Autodesk Inventor part; units mm, degrees
ref_plane "YZ Plane" through (0, 0, 0) normal (1, 0, 0) x (0, 1, 0)
ref_plane "XZ Plane" through (0, 0, 0) normal (0, 1, 0) x (-1, 0, 0)
ref_plane "XY Plane" through (0, 0, 0) normal (0, 0, 1) x (1, 0, 0)
sketch "Sketch1" plane through (0, 0, 0) normal (0, 0, 1) x (1, 0, 0)
  line L0 (0, 0) -> (160, 0)
  line L1 (160, 0) -> (118.589, -154.5481) construction
  line L2 (0, 0) -> (41.411, -154.5481) construction
  line L3 (41.411, -154.5481) -> (118.589, -154.5481)
  circle A0 centre (235.8871, -103.156) radius 80 construction
  line L4 (160, 0) -> (256.5926, -25.8819)
  line L5 (118.589, -154.5481) -> (215.1815, -180.43)
  arc A1 (215.1815, -180.43) -> (256.5926, -25.8819) centre (235.8871, -103.156) ccw
  circle A2 centre (-75.8871, -103.156) radius 80 construction
  line L6 (0, 0) -> (-96.5926, -25.8819)
  line L7 (41.411, -154.5481) -> (-55.1815, -180.43)
  arc A3 (-96.5926, -25.8819) -> (-55.1815, -180.43) centre (-75.8871, -103.156) ccw
  dimension "d0" = 160
  dimension "d1" = 160
  dimension "d2" = 160
  dimension "d3" = 75
  dimension "d4" = 75
  dimension "d5" = 160
  dimension "d6" = 100
  dimension "d7" = 160
  dimension "d9" = 100
extrude "Extrusion1" add sketch "Sketch1" along normal blind 41.5
sketch "Sketch2" plane through (0, 0, 41.5) normal (0, 0, 1) x (1, 0, 0)
  line L0 (-26.5, -133) -> (186.5, -133)
  line L1 (186.5, -133) -> (186.5, -20)
  line L2 (186.5, -20) -> (-26.5, -20)
  line L3 (-26.5, -20) -> (-26.5, -133)
  line L4 (160, 0) -> (0, 0)
  point P0 (80, -20)
  point P1 (80, 0)
  dimension "d12" = 213
  dimension "d13" = 113
  dimension "d14" = 20
extrude "Extrusion2" cut sketch "Sketch2" against normal through all
sketch "Sketch3" plane through (0, 0, 41.5) normal (0, 0, 1) x (1, 0, 0)
  line L0 (-26.5, -133) -> (-26.5, -20) construction
  line L1 (-26.5, -20) -> (186.5, -20) construction
  line L2 (186.5, -20) -> (186.5, -133) construction
  line L3 (186.5, -133) -> (-26.5, -133) construction
  line L4 (-48.0481, 1.5481) -> (-48.0481, -154.5481) construction
  line L5 (-48.0481, -154.5481) -> (208.0481, -154.5481) construction
  line L6 (208.0481, -154.5481) -> (208.0481, 1.5481) construction
  line L7 (208.0481, 1.5481) -> (-48.0481, 1.5481) construction
  line L8 (41.411, -154.5481) -> (118.589, -154.5481) construction
  line L9 (-48.0481, 1.5481) -> (-48.0481, -178.5186) construction
  line L10 (-55.1815, -180.43) -> (41.411, -154.5481) construction
  line L11 (208.0481, 1.5481) -> (208.0481, -178.5186) construction
  line L12 (118.589, -154.5481) -> (215.1815, -180.43) construction
  line L13 (-48.0481, -178.5186) -> (208.0481, -178.5186) construction
  line L14 (-48.0481, 1.5481) -> (208.0481, 1.5481) construction
  line L15 (160, 0) -> (256.5926, -25.8819) construction
  line L16 (208.2963, -12.941) -> (208.0481, -178.5186)
  line L17 (208.2963, -12.941) -> (256.5926, -25.8819)
  line L18 (208.0481, -178.5186) -> (215.1815, -180.43)
  arc A0 (215.1815, -180.43) -> (256.5926, -25.8819) centre (235.8871, -103.156) ccw
  line L19 (208.0481, 1.5481) -> (-166.9519, 1.5481)
  line L20 (-166.9519, 1.5481) -> (-166.9519, -188.4519)
  line L21 (-166.9519, -188.4519) -> (208.0481, -188.4519)
  line L22 (208.0481, -188.4519) -> (208.0481, 1.5481)
  point P0 (0, 0)
  point P1 (80, -154.5481)
  dimension "d17" = 190
  dimension "d18" = 375
extrude "Extrusion3" cut sketch "Sketch3" against normal through all contours L22 L21 L20 L19
sketch "Sketch4" plane through (0, 0, 41.5) normal (0, 0, 1) x (1, 0, 0)
  arc A0 (215.1815, -180.43) -> (256.5926, -25.8819) centre (235.8871, -103.156) ccw
  circle A1 centre (235.8871, -103.156) radius 7
  point P0 (0, 0)
  dimension "d21" = 14
extrude "Extrusion4" cut sketch "Sketch4" against normal through all
sketch "Sketch5" plane through (208.0481, -178.5186, 41.5) normal (-1, 0, 0) x (0, 0, 1)
  line L0 (-41.5, 165.6442) -> (0, 165.6442)
  line L1 (-41.5, 0) -> (-41.5, 165.6442)
  line L2 (0, 0) -> (-41.5, 0)
  line L3 (0, 165.6442) -> (0, 0)
  line L4 (-33, 157.1442) -> (-8.5, 157.1442)
  line L5 (-8.5, 157.1442) -> (-8.5, 8.5)
  line L6 (-8.5, 8.5) -> (-33, 8.5)
  line L7 (-33, 8.5) -> (-33, 157.1442)
  point P0 (-41.5, 178.5186)
  dimension "d24" = 8.5
extrude "Extrusion5" add sketch "Sketch5" along normal blind 13 contours L4 L5 L6 L7
sketch "Sketch6" plane through (208.0481, -170.0186, 8.5) normal (0, 0, -1) x (-1, 0, 0)
  circle A0 centre (8, 74.3221) radius 2.5
  line L0 (0, -8.5) -> (0, 157.1442)
  point P0 (208.0481, 170.0186)
  point P1 (0, 74.3221)
  dimension "d27" = 5
  dimension "d28" = 8
extrude "Extrusion6" cut sketch "Sketch6" against normal through all
sketch "Sketch7" plane through (0, 0, 0) normal (0, 0, -1) x (-1, 0, 0)
  circle A0 centre (-235.8871, -103.156) radius 7
  line L0 (-208.0481, -178.5186) -> (-208.0481, -12.8745)
  line L1 (-208.0481, -12.8745) -> (-256.5926, -25.8819)
  arc A1 (-256.5926, -25.8819) -> (-215.1815, -180.43) centre (-235.8871, -103.156) ccw
  line L2 (-215.1815, -180.43) -> (-208.0481, -178.5186)
  line L3 (-254.522, -33.6093) -> (-216.0481, -23.3003)
  line L4 (-216.0481, -23.3003) -> (-216.0481, -172.38)
  line L5 (-216.0481, -172.38) -> (-217.2521, -172.7026)
  arc A2 (-254.522, -33.6093) -> (-217.2521, -172.7026) centre (-235.8871, -103.156) ccw
  circle A3 centre (-235.8871, -103.156) radius 19
  point P0 (0, 0)
  dimension "d31" = 8
  dimension "d32" = 12
extrude "Extrusion7" cut sketch "Sketch7" against normal through all contours L3 L4 L5 A2
sketch "Sketch8" plane through (0, 0, 0) normal (0, 0, -1) x (-1, 0, 0)
  circle A0 centre (-235.8871, -103.156) radius 7 construction
  circle A1 centre (-235.8871, -103.156) radius 19 construction
  line L0 (-235.8871, -103.156) -> (-159.7277, -103.156) construction
  line L1 (-217.5568, -98.156) -> (-123.6167, -98.156) construction
  line L2 (-217.5568, -108.156) -> (-123.6167, -108.156) construction
  line L3 (-231.052, -84.7815) -> (-184.082, -3.427) construction
  line L4 (-222.3918, -89.7815) -> (-175.4217, -8.427) construction
  line L5 (-249.3823, -89.7815) -> (-296.3524, -8.427) construction
  line L6 (-240.7221, -84.7815) -> (-287.6921, -3.427) construction
  line L7 (-254.2174, -108.156) -> (-348.1575, -108.156) construction
  line L8 (-254.2174, -98.156) -> (-348.1575, -98.156) construction
  line L9 (-240.7221, -121.5305) -> (-287.6921, -202.885) construction
  line L10 (-249.3823, -116.5305) -> (-296.3524, -197.885) construction
  line L11 (-222.3918, -116.5305) -> (-175.4217, -197.885) construction
  line L12 (-231.052, -121.5305) -> (-184.082, -202.885) construction
  line L13 (-216.0481, -23.3003) -> (-216.0481, -172.38) construction
  arc A2 (-254.522, -33.6093) -> (-217.2521, -172.7026) centre (-235.8871, -103.156) ccw construction
  line L14 (-254.522, -33.6093) -> (-216.0481, -23.3003) construction
  line L15 (-216.0481, -172.38) -> (-217.2521, -172.7026) construction
  line L16 (-217.5568, -98.156) -> (-216.0481, -98.156)
  line L17 (-217.5568, -108.156) -> (-216.0481, -108.156)
  line L18 (-222.3918, -116.5305) -> (-216.0481, -127.518)
  line L19 (-231.052, -121.5305) -> (-216.0481, -147.518)
  line L20 (-240.7221, -121.5305) -> (-267.47, -167.8593)
  line L21 (-276.1303, -162.8593) -> (-249.3823, -116.5305)
  line L22 (-254.2174, -108.156) -> (-307.7132, -108.156)
  line L23 (-254.2174, -98.156) -> (-307.7132, -98.156)
  line L24 (-249.3823, -89.7815) -> (-276.1303, -43.4527)
  line L25 (-240.7221, -84.7815) -> (-267.47, -38.4527)
  line L26 (-231.052, -84.7815) -> (-216.0481, -58.7939)
  line L27 (-222.3918, -89.7815) -> (-216.0481, -78.7939)
  line L28 (-216.0481, -58.7939) -> (-216.0481, -78.7939)
  line L29 (-216.0481, -98.156) -> (-216.0481, -108.156)
  line L30 (-216.0481, -127.518) -> (-216.0481, -147.518)
  arc A3 (-267.47, -38.4527) -> (-276.1303, -43.4527) centre (-235.8871, -103.156) ccw
  arc A4 (-307.7132, -98.156) -> (-307.7132, -108.156) centre (-235.8871, -103.156) ccw
  arc A5 (-276.1303, -162.8593) -> (-267.47, -167.8593) centre (-235.8871, -103.156) ccw
  arc A6 (-217.5568, -108.156) -> (-217.5568, -98.156) centre (-235.8871, -103.156) ccw
  arc A7 (-231.052, -121.5305) -> (-222.3918, -116.5305) centre (-235.8871, -103.156) ccw
  arc A8 (-249.3823, -116.5305) -> (-240.7221, -121.5305) centre (-235.8871, -103.156) ccw
  arc A9 (-254.2174, -98.156) -> (-254.2174, -108.156) centre (-235.8871, -103.156) ccw
  arc A10 (-240.7221, -84.7815) -> (-249.3823, -89.7815) centre (-235.8871, -103.156) ccw
  arc A11 (-222.3918, -89.7815) -> (-231.052, -84.7815) centre (-235.8871, -103.156) ccw
  point P0 (0, 0)
  dimension "d36" = 5
  dimension "d37" = 5
  dimension "d40" = 360
extrude "Extrusion8" add sketch "Sketch8" against normal blind 41.5
sketch "Sketch9" plane through (0, 0, 41.5) normal (0, 0, 1) x (1, 0, 0)
  circle A0 centre (235.8871, -103.156) radius 7
  circle A1 centre (235.8871, -103.156) radius 10
  point P0 (0, 0)
  dimension "d46" = 20
extrude "Extrusion9" cut sketch "Sketch9" against normal blind 31
properties part number "Riser Base" material "ABS Plastic"
Verification items for the finished model (mm, model axes). A direction names the side the tool comes from. Coordinates: 2 decimals unless noted, no trailing zeros. Write each loop counter-clockwise with the first axis right and the second up, starting at its lowest first coordinate (ties: lowest second). Pieces come first, ordered by that corner, then holes. Notation, with made-up numbers: (-30, 74) -> (11, 74) arc R26 ccw to (11, 97) -> close; hole circle Ø8 at (56, 23.25). An arc over 180 degrees is marked (long way). One line per item, written item: value. Start each with the question number.
Q1. Cross-section at D-D on y = -153. Enter the section's corners in (x, z).
Q2. Access from +Z, -Z, +X, -X, +Y, -Y to the whole of each face (thin tool, end or side, straight path). Record for faces 5 (the flat face through (203, -97, 8.5)), 6 (the flat face through (216.048, -41, 20)), 7 (the flat face through (203, -95, 33)), 8 (the flat face through (202, -21.374, 21)).
Q3. Cross-section at C-C on z = 36.5. State how many separate pieces and enclosed holes the cut face has, and give its area (3 significant figures).
Q4. Thickness scan on L1, parallel to Y at x = 229.5, z = 6; L2, parallel to Y at x = 268, z = 20; L3, parallel to Y at x = 239, z = 17. Record the ranges inside material, lowest first. Write a range as from..to.
Q5. Go/stop test with flat-tipped pins: P1, Ø4, axis at y = -109.5, z = 29.5, coming from the +X side; P2, Ø4, axis at x = 201.5, z = 15.5, coming from the -Y side; P3, Ø14.5, axis at x = 200.5, y = -97, coming from the -Z side; P4, Ø4, axis at x = 200.05, y = -95.7, coming from the +Z side. Record where each tip stops, or that it passes through.
Q6. Cross-section at B-B on y = -86.5. Enter the section's corners in (x, z).
Q7. Cross-section at A-A on x = 288.5. Enter the section's corners in (y, z), and give its area (3 significant figures).
Q8. Mould release check, pull along X, two halves, no side actions. Record for faces 1 (the flat face through (202, -170.019, 21)), 2 (the cylindrical face through (252.376, -112.597, 20.46)), 3 (the flat face through (281, -98.156, 20)), 4 (the flat face through (211.56, -179.46, 20.46)): pulls with the +X half, pulls with the -X half, needs draft (parallel to the pull), parting line crosses it, or undercut.
Checked values:
1. outline: (195.05, 8.5) -> (208.05, 8.5) -> (208.05, 0) -> (216.05, 0) -> (216.05, 41.5) -> (208.05, 41.5) -> (208.05, 33) -> (195.05, 33) -> close; (258.89, 0) -> (270.44, 0) -> (270.44, 41.5) -> (258.89, 41.5) -> close; (287.84, 0) -> (298.46, 0) -> (298.46, 41.5) -> (287.84, 41.5) -> close
2. face 5: -Z, -X, +Y, -Y
2. face 6: +Z, -Z
2. face 7: +Z, -X, +Y, -Y
2. face 8: +Z, -Z, -X, +Y
3. separate pieces: 1
3. enclosed holes: 7
3. area: 6,410 mm²
4. L1: y = -182.9..-174.87, -124.22..-106.02, -100.29..-82.09, -26.9..-18.62
4. L2: y = -176.43..-148.78, -108.16..-98.16, -57.53..-29.88
4. L3: y = -183.1..-175.09, -121.9..-112.66, -93.65..-84.41, -29.45..-21.17
5. P1: stops at x = 315.77
5. P2: stops at y = -170.02
5. P3: stops at z = 8.5
5. P4: passes through
6. outline: (195.05, 8.5) -> (208.05, 8.5) -> (208.05, 0) -> (216.05, 0) -> (216.05, 41.5) -> (208.05, 41.5) -> (208.05, 33) -> (195.05, 33) -> close; (220.5, 0) -> (251.28, 0) -> (251.28, 41.5) -> (220.5, 41.5) -> close; (305.93, 0) -> (314.13, 0) -> (314.13, 41.5) -> (305.93, 41.5) -> close
7. outline: (-163.42, 0) -> (-152.31, 0) -> (-152.31, 41.5) -> (-163.42, 41.5) -> close; (-108.16, 0) -> (-98.16, 0) -> (-98.16, 41.5) -> (-108.16, 41.5) -> close; (-54, 0) -> (-42.89, 0) -> (-42.89, 41.5) -> (-54, 41.5) -> close
7. area: 1,340 mm²
8. face 1: needs draft
8. face 2: undercut
8. face 3: undercut
8. face 4: pulls with the -X half
